```python
from build123d import *

# Parameters (mm, degrees)
SKETCH4_R             = 68.072
BOSS_EXTRUDE2_DEPTH   = 5.207
SKETCH5_R             = 55.372
CUT_EXTRUDE5_DEPTH    = 6.207
CUT_EXTRUDE11_DEPTH   = 6.207
F_6_32_TAPPED_HOLE1_D = 2.7051


with BuildPart() as part:
    # Sketch4 → Boss-Extrude2 (new body)
    with BuildSketch(Plane.XY):
        Circle(SKETCH4_R)
    extrude(amount=BOSS_EXTRUDE2_DEPTH)

    # Sketch5 → Cut-Extrude5 (cut, through all)
    with BuildSketch(Plane.XY.offset(5.207)):
        Circle(SKETCH5_R)
    extrude(amount=-CUT_EXTRUDE5_DEPTH, mode=Mode.SUBTRACT)

    # Sketch8 → Cut-Extrude11 (cut, through all)
    with BuildSketch(Plane.XY.offset(5.207)):
        Polygon((68.857618113, 29.896397389), (50.084386012, 22.120270044), (51.05640193, 19.773616031), (69.829634031, 27.549743377), align=None)
        Polygon((27.466357594, 62.990983081), (25.119703581, 63.962998999), (24.633695622, 62.789671993), (26.980349635, 61.817656075), align=None)
        Polygon((-25.119703581, 63.962998999), (-27.466357594, 62.990983081), (-26.980349635, 61.817656075), (-24.633695622, 62.789671993), align=None)
        Polygon((-62.990983081, 27.466357594), (-63.962998999, 25.119703581), (-62.789671993, 24.633695622), (-61.817656075, 26.980349635), align=None)
        Polygon((-63.962998999, -25.119703581), (-62.990983081, -27.466357594), (-61.817656075, -26.980349635), (-62.789671993, -24.633695622), align=None)
        Polygon((-27.466357594, -62.990983081), (-25.119703581, -63.962998999), (-24.633695622, -62.789671993), (-26.980349635, -61.817656075), align=None)
        Polygon((25.119703581, -63.962998999), (27.466357594, -62.990983081), (26.980349635, -61.817656075), (24.633695622, -62.789671993), align=None)
        Polygon((62.990983081, -27.466357594), (63.962998999, -25.119703581), (62.789671993, -24.633695622), (61.817656075, -26.980349635), align=None)
    extrude(amount=-CUT_EXTRUDE11_DEPTH, mode=Mode.SUBTRACT)

    # #6-32 Tapped Hole1 (through all)
    with Locations(Plane.XY.offset(5.207)):
        with Locations((61.722, 0), (43.644044748, -43.644044748), (0, -61.722), (-43.644044748, -43.644044748), (-61.722, 0), (-43.644044748, 43.644044748), (0, 61.722), (43.644044748, 43.644044748)):
            Hole(F_6_32_TAPPED_HOLE1_D / 2)


solid = part.part
```
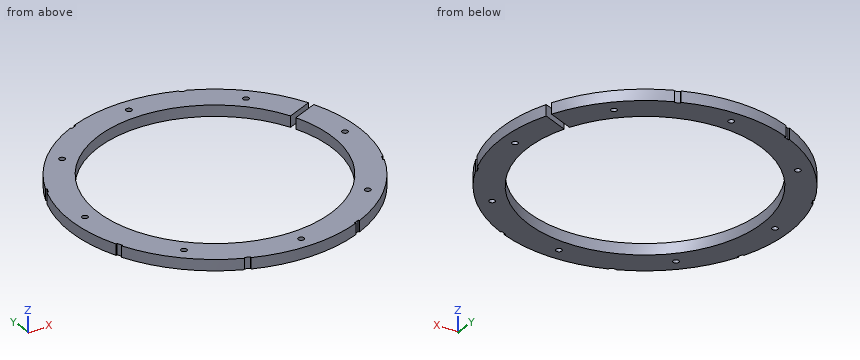
Geometry check sheet. Reference: the model listing, model coordinates, mm. Coordinates: 2 decimals unless noted, no trailing zeros. Loops run counter-clockwise (first coordinate to the right, second up) from the corner with the lowest first, then second, coordinate; pieces in that order, holes last.
Item 1: Sectioned sample at B-B, the plane x = 29. Record the boundary of the cut face in (y, z).
Item 2: Thickness scan on line 1 (Y direction, x = 0, z = 3.2); line 2 (Y direction, x = 62, z = 3.3); line 3 (X direction, y = -1, z = 1.6). Record the ranges inside material, lowest first.
Item 3: Sectioned sample at C-C, the plane z = 1.2. Count the separate pieces of the cut face and the enclosed holes in it, then the cut area to 3 significant figures.
Item 4: Sectioned sample at D-D, the plane y = -57.5. Record the boundary of the cut face in (x, z), then the cut area to 3 significant figures.
Item 5: Go/stop test with flat-tipped pins: pin 1 Ø1.5 at (y, z) = (51.5, 1.5) entering from -X; pin 2 Ø2 at (y, z) = (-29.5, 1) entering from -X; pin 3 Ø1 at (y, z) = (2, 3.5) entering from +X; pin 4 Ø3.5 at (x, y) = (-43.64, 43.64) entering from -Z. Record where each tip stops, or that it passes through.
Item 6: Sectioned sample at A-A, the plane x = -48.5. Record the boundary of the cut face in (y, z), then the cut area to 3 significant figures.
Check result:
1. outline: (-61.59, 0) - (-47.17, 0) - (-47.17, 5.21) - (-61.59, 5.21) - close; (47.17, 0) - (61.59, 0) - (61.59, 5.21) - (47.17, 5.21) - close
2. line 1: y = -68.07 to -63.07, -60.37 to -55.37, 55.37 to 60.37, 63.07 to 68.07
2. line 2: y = -28.1 to -27.06, -26.54 to -1.32, 1.32 to 24.31, 27.06 to 28.1
2. line 3: x = -68.06 to -62.63, -60.81 to -55.36, 55.36 to 60.81, 62.63 to 68.06
3. separate pieces: 1
3. enclosed holes: 8
3. area: 4,840 mm2
4. outline: (-36.44, 0) - (36.44, 0) - (36.44, 5.21) - (-36.44, 5.21) - close
4. area: 379 mm2
5. pin 1: stops at x = -45.37
5. pin 2: stops at x = -61.82
5. pin 3: stops at x = 68.06
5. pin 4: stops at z = 0
6. outline: (-47.77, 0) - (-26.72, 0) - (-26.72, 5.21) - (-47.77, 5.21) - close; (26.72, 0) - (47.77, 0) - (47.77, 5.21) - (26.72, 5.21) - close
6. area: 219 mm2
